Design review of the part shown in the three views and the two pictorial views. Dimensions are in mm from the part's minimum x, y and z. A direction names the side the tool comes from. Round coordinates to 2 decimals unless told otherwise and drop trailing zeros. Loops run counter-clockwise (first coordinate to the right, second up) from the corner with the lowest first, then second, coordinate; pieces in that order, holes last. Notation, with made-up numbers: (83.5, -22) -> (139.5, -22) arc R16 ccw to (139.5, -9) -> close; hole circle Ø7 at (63.5, 47.5). An arc over 180 degrees is marked (long way). Use CSV: the item, a comma, the result in double quotes. Start each with the question number.
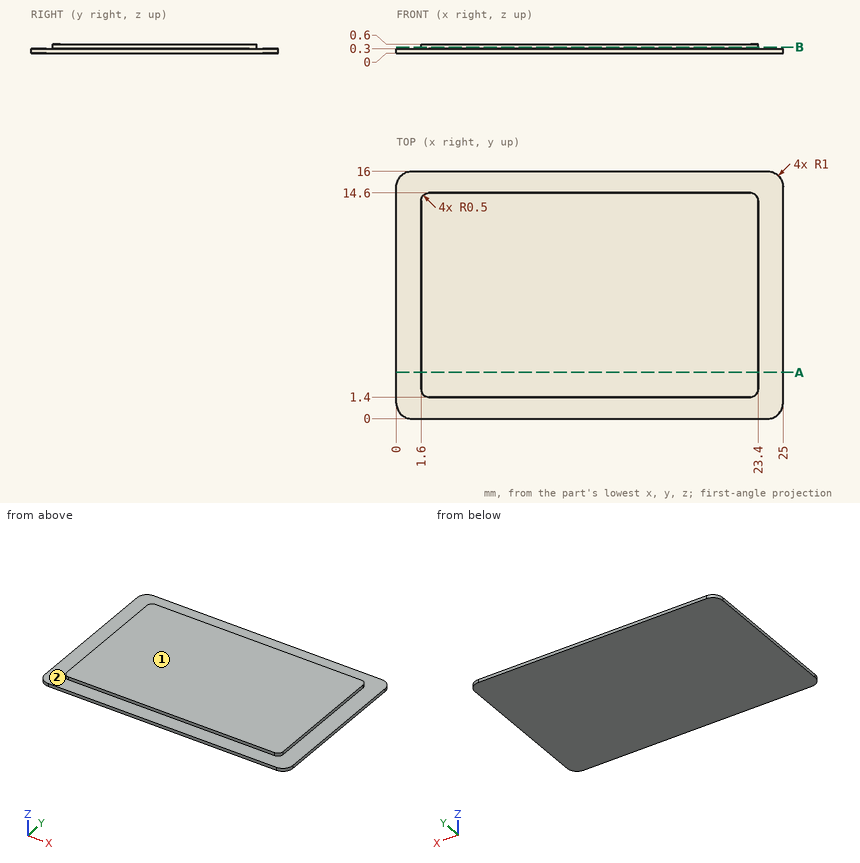
1. For line 1 along Y through (x, z) = (18, 0.4); line 2 along X through (y, z) = (6.5, 0.5); line 3 along Z through (x, y) = (23.5, 8.75), list the stretches that pass through material, from the lowest coordinate up. Write a range as from..to.
2. For the marked faces 1 and 2, list the 3-axis set-ups (+Z, -Z, +X, -X, +Y, -Y) from which the entire face can be reached by the end or side of a thin tool; tool diameter is ignored.
3. Take a section at A-A, the plane y = 3. Give the boundary of the cut face in (x, z).
4. Take a section at B-B, the plane z = 0.4. Give the boundary of the cut face in (x, y).
Results:
1,line 1,"1.4..14.6"
1,line 2,"1.6..23.4"
1,line 3,"0..0.3"
2,face 1,"+Z, +X, -X, +Y, -Y"
2,face 2,"+Z"
3,outline,"(0, 0) -> (25, 0) -> (25, 0.3) -> (23.4, 0.3) -> (23.4, 0.6) -> (1.6, 0.6) -> (1.6, 0.3) -> (0, 0.3) -> close"
4,outline,"(1.6, 1.9) arc R0.5 ccw to (2.1, 1.4) -> (22.9, 1.4) arc R0.5 ccw to (23.4, 1.9) -> (23.4, 14.1) arc R0.5 ccw to (22.9, 14.6) -> (2.1, 14.6) arc R0.5 ccw to (1.6, 14.1) -> close"
